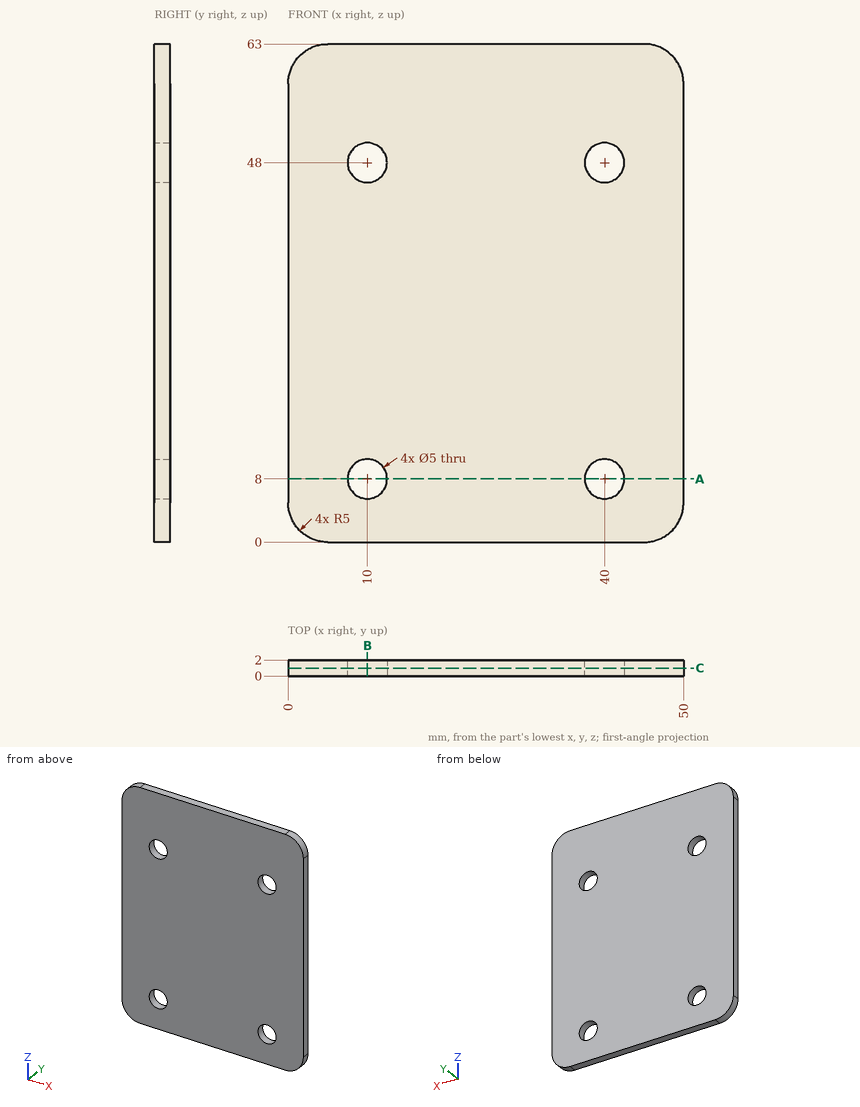
For this review, use the dimensioned drawing (mm, ordinates from the lowest corner) and the shaded views. Coordinates: 2 decimals unless noted, no trailing zeros. Loops run counter-clockwise (first coordinate to the right, second up) from the corner with the lowest first, then second, coordinate; pieces in that order, holes last.
1. Insertion check: P1, Ø4.5, axis at x = 40, z = 8, coming from the -Y side. The pin has a flat end and moves straight along its axis. Give the tip position at first contact, or say it passes through.
2. For line 1 (Z direction, x = 10, y = 0.7); line 2 (Z direction, x = 42, y = 1.3); line 3 (X direction, y = 1.2, z = 6.5), list the stretches that pass through material, from the lowest coordinate up.
3. Add section B-B, the plane x = 10. Give the boundary of the cut face in (y, z).
4. Add section A-A, the plane z = 8. Give the boundary of the cut face in (x, y).
5. Add section C-C, the plane y = 1. Give the boundary of the cut face in (x, z).
Result:
1. P1: passes through
2. line 1: z = 0 to 5.5, 10.5 to 45.5, 50.5 to 63
2. line 2: z = 0 to 6.5, 9.5 to 46.5, 49.5 to 63
2. line 3: x = 0 to 8, 12 to 38, 42 to 50
3. outline: (0, 0) - (2, 0) - (2, 5.5) - (0, 5.5) - close; (0, 10.5) - (2, 10.5) - (2, 45.5) - (0, 45.5) - close; (0, 50.5) - (2, 50.5) - (2, 63) - (0, 63) - close
4. outline: (0, 0) - (7.5, 0) - (7.5, 2) - (0, 2) - close; (12.5, 0) - (37.5, 0) - (37.5, 2) - (12.5, 2) - close; (42.5, 0) - (50, 0) - (50, 2) - (42.5, 2) - close
5. outline: (0, 5) arc R5 ccw to (5, 0) - (45, 0) arc R5 ccw to (50, 5) - (50, 58) arc R5 ccw to (45, 63) - (5, 63) arc R5 ccw to (0, 58) - close; hole circle Ø5 at (10, 8); hole circle Ø5 at (10, 48); hole circle Ø5 at (40, 8); hole circle Ø5 at (40, 48)
